from build123d import *

# Parameters (mm, degrees)
ESQUISSE1_W             = 125
ESQUISSE1_H             = 60
ESQUISSE1_R             = 1.5
BOSS_EXTRU_1_DEPTH      = 6
ESQUISSE2_W             = 40
ESQUISSE2_H             = 25
ESQUISSE2_W_2           = 35
ESQUISSE2_H_2           = 1
ENL_V_MAT_EXTRU_1_DEPTH = 6


with BuildPart() as part:
    # Esquisse1 → Boss.-Extru.1 (new body)
    with BuildSketch(Plane.XY):
        with Locations((16.823229439, -0.568627451)):
            Rectangle(ESQUISSE1_W, ESQUISSE1_H)
        with Locations((-31.676770561, 24.431372549)):
            Circle(ESQUISSE1_R, mode=Mode.SUBTRACT)
        with Locations((-21.676770561, 24.431372549)):
            Circle(ESQUISSE1_R, mode=Mode.SUBTRACT)
    extrude(amount=BOSS_EXTRU_1_DEPTH)

    # Esquisse2 → Enlèv. mat.-Extru.1 (cut)
    with BuildSketch(Plane.XY.offset(6)):
        with Locations((-25.676770561, -18.068627451)):
            Rectangle(ESQUISSE2_W, ESQUISSE2_H)
        with Locations((-28.176770561, 28.931372549)):
            Rectangle(ESQUISSE2_W_2, ESQUISSE2_H_2)
    extrude(amount=-ENL_V_MAT_EXTRU_1_DEPTH, mode=Mode.SUBTRACT)


solid = part.part
Part model, mm, in its own coordinate system. A direction names the side the tool comes from. Round coordinates to 2 decimals unless told otherwise and drop trailing zeros. Write each loop counter-clockwise with the first axis right and the second up, starting at its lowest first coordinate (ties: lowest second). Pieces come first, ordered by that corner, then holes. Notation, with made-up numbers: M -10,38.5 L 19,38.5 A18 ccw 19,55.5 Z; hole C 2.25,27.5 d1. An arc over 180 degrees is marked long. Return JSON: item names as keys, results as strings. Group by question number.
(1) Pin check, flat tips, straight feed: pin 1 Ø0.8 at (y, z) = (29, 2) entering from -X; pin 2 Ø1.5 at (x, z) = (-9, 3) entering from -Y; pin 3 Ø3 at (y, z) = (-16.5, 4) entering from -X. Stop position of each tip, or through.
(2) Two-plate mould, pull along Y, no slides. Class faces 4 (the face through (-45.677, 11, 3)), 5 (the face through (34, 29.431, 3)), 6 (the face through (-22.87, 23.52, 2.96)): +Y half, -Y half, draft (parallel to the pull), parting line (faces both ways), or undercut.
(3) Which spindle directions (+Z, -Z, +X, -X, +Y, -Y) get a long thin tool onto all of the face, cutting with end or side? Do faces 1 (the face through (-26, -5.569, 3)), 2 (the face through (-28, 28.431, 3)), 3 (the face through (79.323, -1, 3)). Say none if no direction does.
(4) Saw through at A-A on z = 1.1. Write the cut outline in (x, y), then the cut area to 3 significant figures.
(5) Drill centre lines: probe 1 along Y at (x, z) = (-18.5, 5.25); probe 2 along X at (y, z) = (-21, 1.9); probe 3 along Y at (x, z) = (-7, 5.75). Where is each one in solid material? Low to high.
(6) Saw through at B-B on y = -22.5. Write the cut outline in (x, z), then the cut area to 3 significant figures.
(7) Saw through at C-C on x = -26. Write the cut outline in (y, z), then the cut area to 3 significant figures.
Returned:
{
 "1": {"pin 1": "x = -10.68", "pin 2": "y = -5.57", "pin 3": "x = -5.68"},
 "2": {"face 4": "draft", "face 5": "+Y half", "face 6": "undercut"},
 "3": {"face 1": "+Z, -Z, -X, -Y", "face 2": "+Z, -Z, -X, +Y", "face 3": "+Z, -Z, +X, +Y, -Y"},
 "4": {"outline": "M -45.68,-5.57 L -5.68,-5.57 L -5.68,-30.57 L 79.32,-30.57 L 79.32,29.43 L -10.68,29.43 L -10.68,28.43 L -45.68,28.43 Z; hole C -31.68,24.43 d3; hole C -21.68,24.43 d3", "area": "6,450 mm²"},
 "5": {"probe 1": "-5.57 to 28.43", "probe 2": "-5.68 to 79.32", "probe 3": "-5.57 to 29.43"},
 "6": {"outline": "M -5.68,0 L 79.32,0 L 79.32,6 L -5.68,6 Z", "area": "510 mm²"},
 "7": {"outline": "M -5.57,0 L 28.43,0 L 28.43,6 L -5.57,6 Z", "area": "204 mm²"}
}
